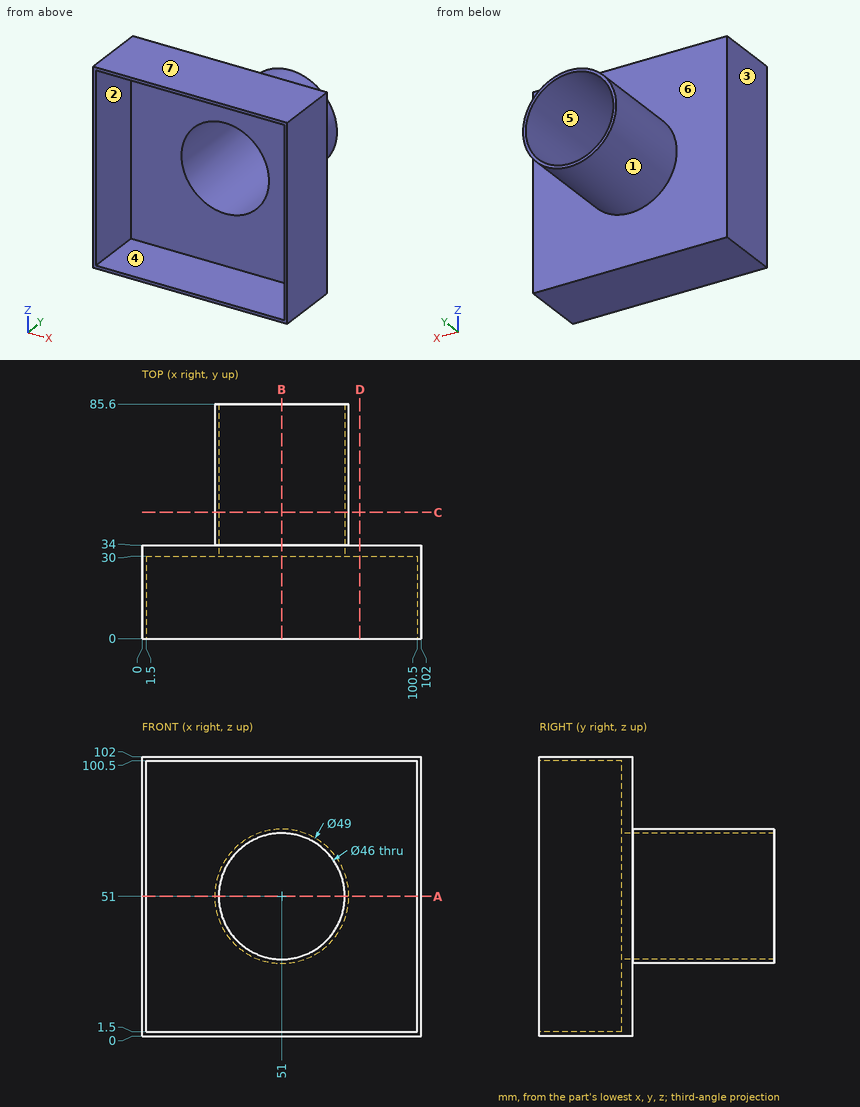
Check sheet for the drawn part. Datum: minimum x, y, z corner. Units: mm. A direction names the side the tool comes from. Give positions to 0.01 mm unless a question says otherwise; leave off trailing zeros. Write each loop counter-clockwise with the first axis right and the second up, starting at its lowest first coordinate (ties: lowest second). Pieces come first, ordered by that corner, then holes.
(1) Cross-section at A-A (z = 51). Enter the section's corners in (x, y), plus the area to 3 significant figures.
(2) Cross-section at C-C (y = 46). Enter the section's corners in (x, z), plus the area to 3 significant figures.
(3) Gauge pin test, flat ends, axial feed: pin 1 (12 mm diameter, centred on y = 31, z = 89.5, fed in from -X); pin 2 (3 mm diameter, centred on x = 51.5, y = 48.5, fed in from +Z); pin 3 (6 mm diameter, centred on x = 25, z = 24.5, fed in from +Y); pin 4 (6 mm diameter, centred on x = 42.5, y = 46, fed in from +Z). Record the tip position at first contact, or that the pin passes through.
(4) Cross-section at D-D (x = 79.5). Enter the section's corners in (y, z).
(5) Mould release check, pull along Z, two halves, no side actions. Record for the marked faces 4, 5, 6 and 7: +Z half, -Z half, draft (parallel to the pull), parting line (faces both ways), or undercut.
(6) Material ranges on line 1 (X direction, y = 16, z = 50.5); line 2 (Z direction, x = 51, y = 46.5); line 3 (Y direction, x = 42.5, z = 81), recorded low to high.
(7) Access from +Z, -Z, +X, -X, +Y, -Y to the whole of each face (thin tool, end or side, straight path). Record for the marked faces 1, 2 and 3.
(8) Cross-section at B-B (x = 51). Enter the section's corners in (y, z), plus the area to 3 significant figures.
Worked out:
1. outline: (0, 0) - (1.5, 0) - (1.5, 30) - (28, 30) - (28, 85.6) - (26.5, 85.6) - (26.5, 34) - (0, 34) - close; (74, 30) - (100.5, 30) - (100.5, 0) - (102, 0) - (102, 34) - (75.5, 34) - (75.5, 85.6) - (74, 85.6) - close
1. area: 469 mm2
2. outline: circle Ø49 at (51, 51); hole circle Ø46 at (51, 51)
2. area: 224 mm2
3. pin 1: stops at x = 0
3. pin 2: stops at z = 75.5
3. pin 3: stops at y = 34
3. pin 4: stops at z = 74.87
4. outline: (0, 0) - (34, 0) - (34, 102) - (0, 102) - (0, 100.5) - (30, 100.5) - (30, 1.5) - (0, 1.5) - close
5. face 4: undercut
5. face 5: undercut
5. face 6: draft
5. face 7: +Z half
6. line 1: x = 0 to 1.5, 100.5 to 102
6. line 2: z = 26.5 to 28, 74 to 75.5
6. line 3: y = 30 to 34
7. face 1: +Y
7. face 2: -Y
7. face 3: +Z, -Z, -X, +Y, -Y
8. outline: (0, 0) - (34, 0) - (34, 26.5) - (85.6, 26.5) - (85.6, 28) - (30, 28) - (30, 1.5) - (0, 1.5) - close; (0, 100.5) - (30, 100.5) - (30, 74) - (85.6, 74) - (85.6, 75.5) - (34, 75.5) - (34, 102) - (0, 102) - close
8. area: 469 mm2
